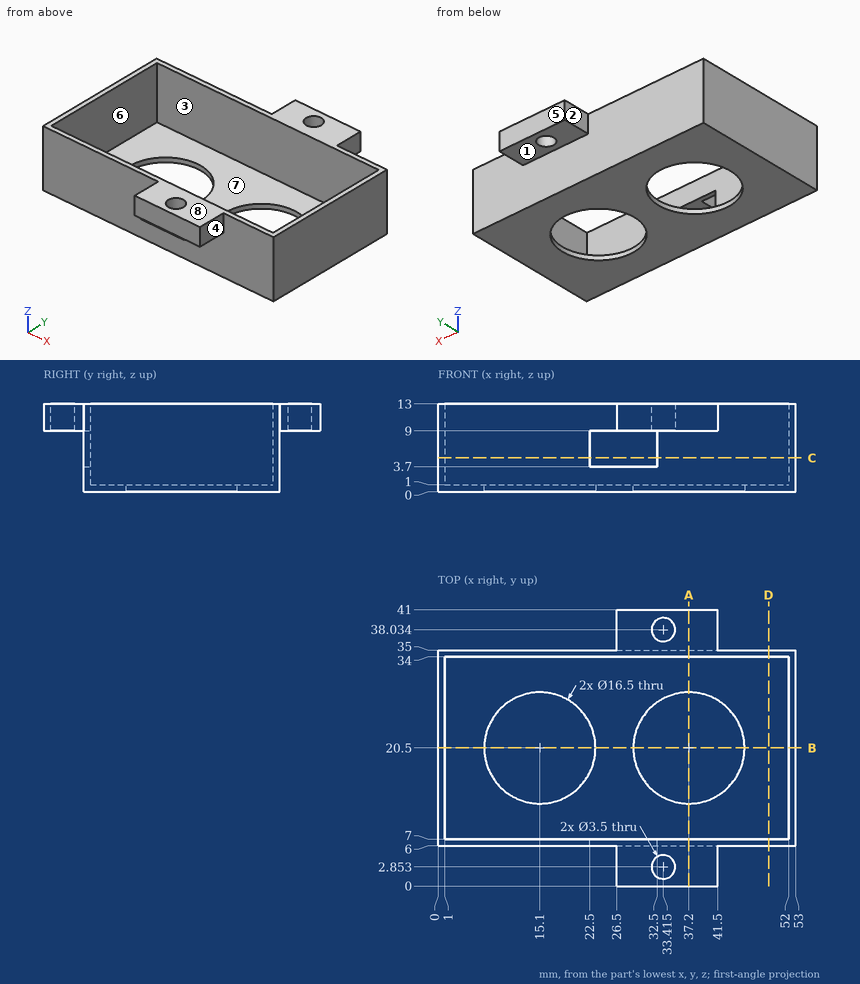
Job drawing, mm, ordinate dimensions from the low corner. One solid piece. A direction names the side the tool comes from. Coordinates: 2 decimals unless noted, no trailing zeros. Order: outer loops, then holes, each group sorted by start corner. A loop starts at its lowest first (then second) coordinate and runs counter-clockwise, first axis right, second up. Notation, with made-up numbers: (-0.5, 31.25) - (32.5, 31.25) arc R9 cw to (32.5, 41.25) - close; hole circle Ø10 at (74.25, -14.75). An arc over 180 degrees is marked (long way). Return JSON: item names as keys, results as strings. Group by question number.
1) Tool access for the marked faces 1, 2, 3 and 4: list every direction of +Z, -Z, +X, -X, +Y, -Y with a clear straight run to the whole face (end or side of a thin tool).
2) Flat gauge pins, fed straight in: P1, Ø4, axis at x = 37, y = 29.5, coming from the +Z side; P2, Ø1, axis at x = 43.5, z = 2.5, coming from the -Y side; P3, Ø3, axis at y = 2, z = 10.5, coming from the +X side; P4, Ø3, axis at x = 33.41, y = 38.03, coming from the -Z side. Where does each tip first touch, or does it go through?
3) Mould opens along Y. For the marked faces 5, 6, 7 and 8 say: released by +Y, released by -Y, zero draft, split by the parting line, or undercut.
4) Saw through at C-C, the plane z = 5. Write the cut outline in (x, y), plus the area to 3 significant figures.
5) Probe line 1 (Y direction, x = 50, z = 1.5); line 2 (X direction, y = 19, z = 9.25); line 3 (Z direction, x = 13, y = 31). List the from-to ranges inside material, lowest first. Write a range as from..to.
6) Saw through at D-D, the plane x = 49. Write the cut outline in (y, z).
7) Saw through at B-B, the plane y = 20.5. Write the cut outline in (x, z).
8) Saw through at A-A, the plane x = 37.2. Write the cut outline in (y, z).
Values found:
{
 "1": {"face 1": "-Z, +X, -X, +Y", "face 2": "+Z, -Z, -X, +Y", "face 3": "+Z", "face 4": "+Z, -Z, +X, -Y"},
 "2": {"P1": "stops at z = 1", "P2": "stops at y = 6", "P3": "stops at x = 41.5", "P4": "passes through"},
 "3": {"face 5": "released by +Y", "face 6": "undercut", "face 7": "undercut", "face 8": "zero draft"},
 "4": {"outline": "(0, 6) - (22.5, 6) - (22.5, 7) - (1, 7) - (1, 34) - (52, 34) - (52, 7) - (32.5, 7) - (32.5, 6) - (53, 6) - (53, 35) - (0, 35) - close", "area": "150 mm²"},
 "5": {"line 1": "y = 6..7, 34..35", "line 2": "x = 0..1, 52..53", "line 3": "z = 0..1"},
 "6": {"outline": "(6, 0) - (35, 0) - (35, 13) - (34, 13) - (34, 1) - (7, 1) - (7, 13) - (6, 13) - close"},
 "7": {"outline": "(0, 0) - (6.85, 0) - (6.85, 1) - (1, 1) - (1, 13) - (0, 13) - close; (23.35, 0) - (28.95, 0) - (28.95, 1) - (23.35, 1) - close; (45.45, 0) - (53, 0) - (53, 13) - (52, 13) - (52, 1) - (45.45, 1) - close"},
 "8": {"outline": "(0, 9) - (6, 9) - (6, 0) - (12.25, 0) - (12.25, 1) - (7, 1) - (7, 13) - (0, 13) - close; (28.75, 0) - (35, 0) - (35, 9) - (41, 9) - (41, 13) - (34, 13) - (34, 1) - (28.75, 1) - close"}
}
